Geometry check sheet. Reference: drawing and pictorial views, mm from the part's lowest x, y, z. A direction names the side the tool comes from. Round coordinates to 2 decimals unless told otherwise and drop trailing zeros. Order: outer loops, then holes, each group sorted by start corner. A loop starts at its lowest first (then second) coordinate and runs counter-clockwise, first axis right, second up.
(1) Sectioned sample at C-C (x = 17.5). Record the boundary of the cut face in (y, z).
(2) Sectioned sample at B-B (z = 10). Record the boundary of the cut face in (x, y).
(3) Sectioned sample at A-A (x = 28.5). Record the boundary of the cut face in (y, z).
(4) Go/stop test with flat-tipped pins: pin 1 (14 mm diameter, centred on x = 13, y = 10, fed in from +Z); pin 2 (6 mm diameter, centred on x = 5, z = 10, fed in from +Y). Record where each tip stops, or that it passes through.
(5) Set-up check for the marked faces 1 and 2: record each of +Z, -Z, +X, -X, +Y, -Y from which the full face is reachable in a straight line by a thin tool's end or side.
(6) Sectioned sample at D-D (z = 8.25). Record the boundary of the cut face in (x, y) (1 decimal).
(7) Material ranges on line 1 along X through (y, z) = (0.65, 10); line 2 along Z through (x, y) = (30, 1.2); line 3 along Z through (x, y) = (21, 13.5), recorded low to high.
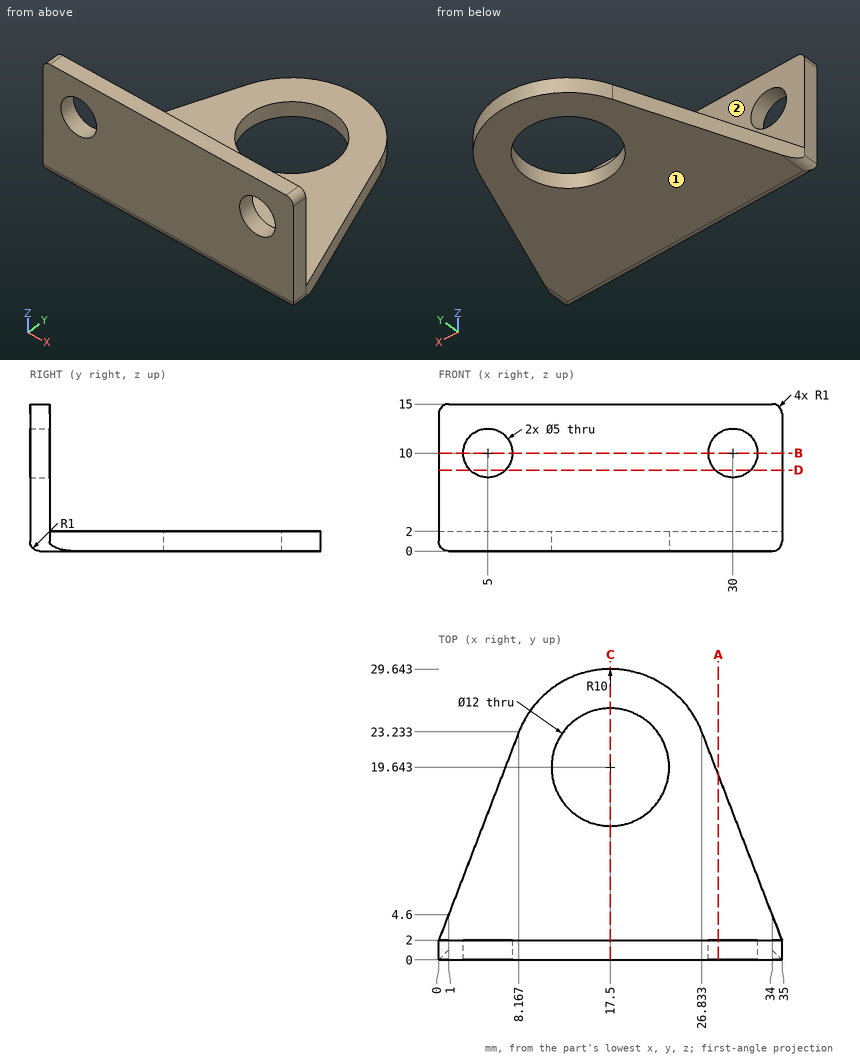
Answer below:
1. outline: (0, 1) arc R1 ccw to (1, 0) - (13.64, 0) - (13.64, 2) - (2, 2) - (2, 15) - (0, 15) - close; (25.64, 0) - (29.64, 0) - (29.64, 2) - (25.64, 2) - close
2. outline: (0, 0) - (2.5, 0) - (2.5, 2) - (0, 2) - close; (7.5, 0) - (27.5, 0) - (27.5, 2) - (7.5, 2) - close; (32.5, 0) - (35, 0) - (35, 2) - (32.5, 2) - close
3. outline: (0, 1) arc R1 ccw to (1, 0) - (18.9, 0) - (18.9, 2) - (2, 2) - (2, 8) - (0, 8) - close; (0, 12) - (2, 12) - (2, 15) - (0, 15) - close
4. pin 1: stops at z = 2
4. pin 2: stops at y = 2
5. face 1: -Z, +X, -X, +Y, -Y
5. face 2: +Z, +X, -X, +Y
6. outline: (0, 0) - (3.2, 0) - (3.2, 2) - (0, 2) - close; (6.8, 0) - (28.2, 0) - (28.2, 2) - (6.8, 2) - close; (31.8, 0) - (35, 0) - (35, 2) - (31.8, 2) - close
7. line 1: x = 0 to 2.5, 7.5 to 27.5, 32.5 to 35
7. line 2: z = 0 to 7.5, 12.5 to 15
7. line 3: z = 0 to 2
